```python
from build123d import *

# Parameters (mm, degrees)
ESQUISSE1_W             = 10
ESQUISSE1_H             = 6
BOSS_EXTRU_1_DEPTH      = 6
ESQUISSE2_R             = 12.5
ESQUISSE2_R_2           = 7.5
ENL_V_MAT_EXTRU_1_DEPTH = 6
ESQUISSE4_R             = 4
ENL_V_MAT_EXTRU_2_DEPTH = 6
CONG_1_R                = 10


with BuildPart() as part:
    # Esquisse1 → Boss.-Extru.1 (new body)
    with BuildSketch(Plane(origin=(0, 0, 0), x_dir=(1, 0, 0), z_dir=(0, 1, 0))):
        Polygon((-14.271309642, 11), (-14.271309642, 359), (25.728690358, 359), (25.728690358, 370), (67, 370), (67, 0), (25.728690358, 0), (25.728690358, 11), align=None)
        with Locations((44, 362)):
            Rectangle(ESQUISSE1_W, ESQUISSE1_H, mode=Mode.SUBTRACT)
        with Locations((44, 8)):
            Rectangle(ESQUISSE1_W, ESQUISSE1_H, mode=Mode.SUBTRACT)
    extrude(amount=BOSS_EXTRU_1_DEPTH)

    # Esquisse2 → Enl_v. mat.-Extru.1 (cut)
    with BuildSketch(Plane(origin=(0, 6, 0), x_dir=(1, 0, 0), z_dir=(0, 1, 0))):
        with Locations(Location((51, 315, 0), (0, 0, 270))):
            Circle(ESQUISSE2_R)
        with Locations(Location((51, 282.5, 0), (0, 0, 270))):
            Circle(ESQUISSE2_R)
        with Locations(Location((51, 250, 0), (0, 0, 270))):
            Circle(ESQUISSE2_R)
        with Locations(Location((51, 217.5, 0), (0, 0, 270))):
            Circle(ESQUISSE2_R)
        with Locations(Location((51, 185, 0), (0, 0, 270))):
            Circle(ESQUISSE2_R)
        with Locations(Location((51, 152.5, 0), (0, 0, 270))):
            Circle(ESQUISSE2_R)
        with Locations(Location((51, 120, 0), (0, 0, 270))):
            Circle(ESQUISSE2_R)
        with Locations(Location((51, 87.5, 0), (0, 0, 270))):
            Circle(ESQUISSE2_R)
        with Locations(Location((51, 55, 0), (0, 0, 270))):
            Circle(ESQUISSE2_R)
        with Locations(Location((21, 315, 0), (0, 0, 270))):
            Circle(ESQUISSE2_R_2)
        with Locations(Location((21, 282.5, 0), (0, 0, 270))):
            Circle(ESQUISSE2_R_2)
        with Locations(Location((21, 250, 0), (0, 0, 270))):
            Circle(ESQUISSE2_R_2)
        with Locations(Location((21, 217.5, 0), (0, 0, 270))):
            Circle(ESQUISSE2_R_2)
        with Locations(Location((21, 185, 0), (0, 0, 270))):
            Circle(ESQUISSE2_R_2)
        with Locations(Location((21, 152.5, 0), (0, 0, 270))):
            Circle(ESQUISSE2_R_2)
        with Locations(Location((21, 120, 0), (0, 0, 270))):
            Circle(ESQUISSE2_R_2)
        with Locations(Location((21, 87.5, 0), (0, 0, 270))):
            Circle(ESQUISSE2_R_2)
        with Locations(Location((21, 55, 0), (0, 0, 270))):
            Circle(ESQUISSE2_R_2)
    extrude(amount=-ENL_V_MAT_EXTRU_1_DEPTH, mode=Mode.SUBTRACT)

    # Esquisse4 → Enl_v. mat.-Extru.2 (cut)
    with BuildSketch(Plane(origin=(0, 6, 0), x_dir=(1, 0, 0), z_dir=(0, 1, 0))):
        with Locations(Location((54.886501567, 22, 0), (0, 0, 270))):
            Circle(ESQUISSE4_R)
        with Locations(Location((42.886501567, 22, 0), (0, 0, 270))):
            Circle(ESQUISSE4_R)
        with Locations(Location((30.886501567, 22, 0), (0, 0, 270))):
            Circle(ESQUISSE4_R)
        with Locations(Location((42.886501567, 34, 0), (0, 0, 270))):
            Circle(ESQUISSE4_R)
        with Locations(Location((30.886501567, 34, 0), (0, 0, 270))):
            Circle(ESQUISSE4_R)
        with Locations(Location((54.886501567, 34, 0), (0, 0, 270))):
            Circle(ESQUISSE4_R)
        with Locations(Location((54.886501567, 336, 0), (0, 0, 90))):
            Circle(ESQUISSE4_R)
        with Locations(Location((30.886501567, 336, 0), (0, 0, 90))):
            Circle(ESQUISSE4_R)
        with Locations(Location((42.886501567, 336, 0), (0, 0, 90))):
            Circle(ESQUISSE4_R)
        with Locations(Location((30.886501567, 348, 0), (0, 0, 90))):
            Circle(ESQUISSE4_R)
        with Locations(Location((42.886501567, 348, 0), (0, 0, 90))):
            Circle(ESQUISSE4_R)
        with Locations(Location((54.886501567, 348, 0), (0, 0, 90))):
            Circle(ESQUISSE4_R)
    extrude(amount=-ENL_V_MAT_EXTRU_2_DEPTH, mode=Mode.SUBTRACT)

    # Cong_1
    cong_1_edges = [part.edges().sort_by_distance(p)[0] for p in [
        (67, 3, 0),
        (67, 3, -370),
    ]]
    fillet(cong_1_edges, radius=CONG_1_R)


solid = part.part
```
Can you work these out from the model? Positions are in its coordinate system, mm. A direction names the side the tool comes from. Give positions to 0.01 mm unless a question says otherwise; leave off trailing zeros. Loops run counter-clockwise (first coordinate to the right, second up) from the corner with the lowest first, then second, coordinate; pieces in that order, holes last. Notation, with made-up numbers: M -15,25 L -7,25 A29 cw -7,49 Z; hole C 70.5,35.25 d5. An arc over 180 degrees is marked long. Answer in a Markdown table with one row per item.
1. Suppose I cut it at C-C on x = -7. Write out the boundary of the cut face in (y, z), plus the area to 3 significant figures.
Taken from the geometry:
| item | result |
|---|---|
| outline | M 0,-359 L 6,-359 L 6,-11 L 0,-11 Z |
| area | 2,090 mm² |
2. Suppose I cut it at B-B on z = -282.5. Write out the boundary of the cut face in (x, y), plus the area to 3 significant figures.
Taken from the geometry:
| item | result |
|---|---|
| outline | M -14.27,0 L 13.5,0 L 13.5,6 L -14.27,6 Z; M 28.5,0 L 38.5,0 L 38.5,6 L 28.5,6 Z; M 63.5,0 L 67,0 L 67,6 L 63.5,6 Z |
| area | 248 mm² |
3. Suppose I cut it at A-A on z = -22. Write out the boundary of the cut face in (x, y).
Taken from the geometry:
| item | result |
|---|---|
| outline | M -14.27,0 L 26.89,0 L 26.89,6 L -14.27,6 Z; M 34.89,0 L 38.89,0 L 38.89,6 L 34.89,6 Z; M 46.89,0 L 50.89,0 L 50.89,6 L 46.89,6 Z; M 58.89,0 L 67,0 L 67,6 L 58.89,6 Z |
4. If I drill on line 1 along X through (y, z) = (2.6, -348); line 2 along X through (y, z) = (3.9, -282.5); line 3 along X through (y, z) = (0.9, -158), over which ranges is the centre line in solid material (lowest first)?
Taken from the geometry:
| item | result |
|---|---|
| line 1 | x = -14.27 to 26.89, 34.89 to 38.89, 46.89 to 50.89, 58.89 to 67 |
| line 2 | x = -14.27 to 13.5, 28.5 to 38.5, 63.5 to 67 |
| line 3 | x = -14.27 to 15.9, 26.1 to 39.78, 62.22 to 67 |
5. Suppose I cut it at D-D on x = 21. Count the separate pieces of the cut face and the enclosed holes in it, plus the area to 3 significant figures.
Taken from the geometry:
| item | result |
|---|---|
| separate pieces | 10 |
| enclosed holes | 0 |
| area | 1,280 mm² |
6. Which directions (+Z, -Z, +X, -X, +Y, -Y) give clear straight access to the entire face, cutting with the end or side of a thin tool? Please do faces 5 (the flat face through (6, 3, -11)), 6 (the flat face through (49, 3, -8)), 7 (the flat face through (67, 3, -187)).
Taken from the geometry:
| item | result |
|---|---|
| face 5 | +Z, -X, +Y, -Y |
| face 6 | +Y, -Y |
| face 7 | +Z, -Z, +X, +Y, -Y |
7. Thinking about a two-plate mould opening in X: for faces 1 (the flat face through (41, 3, -370)), 2 (the cylindrical face through (54.755, 3.042, -303.077)), 3 (the cylindrical face through (38.982, 3.042, -34.867)), 4 (the cylindrical face through (63.99, 3.04, -367.15)), which applies, released by +X, released by -X, zero draft, split by the parting line, or undercut?
Taken from the geometry:
| item | result |
|---|---|
| face 1 | zero draft |
| face 2 | undercut |
| face 3 | undercut |
| face 4 | released by +X |
